from build123d import *

# Parameters (mm, degrees)
SKETCH1_W           = 15.8
SKETCH1_H           = 4
SKETCH1_W_2         = 2.7
SKETCH1_H_2         = 2.7
BOSS_EXTRUDE1_DEPTH = 7.65
SKETCH2_W           = 15.8
SKETCH2_H           = 4
SKETCH2_W_2         = 1.8
SKETCH2_H_2         = 1.8
BOSS_EXTRUDE2_DEPTH = 1
SKETCH3_W           = 2.45
SKETCH3_H           = 2.45
SKETCH3_W_2         = 1.8
SKETCH3_H_2         = 1.8
BOSS_EXTRUDE3_DEPTH = 6.35
SKETCH4_W           = 4.65
SKETCH4_H           = 0.65
SKETCH4_W_2         = 15.8
BOSS_EXTRUDE4_DEPTH = 1
SKETCH5_W           = 1
SKETCH5_H           = 1
SKETCH5_W_2         = 0.4
BOSS_EXTRUDE5_DEPTH = 2.5


with BuildPart() as part:
    # Sketch1 → Boss-Extrude1 (new body)
    with BuildSketch(Plane(origin=(0, 0, 0), x_dir=(1, 0, 0), z_dir=(0, 1, 0))):
        Rectangle(SKETCH1_W, SKETCH1_H)
        Rectangle(SKETCH1_W_2, SKETCH1_H_2, mode=Mode.SUBTRACT)
        with Locations((3, 0)):
            Rectangle(SKETCH1_W_2, SKETCH1_H_2, mode=Mode.SUBTRACT)
        with Locations((6, 0)):
            Rectangle(SKETCH1_W_2, SKETCH1_H_2, mode=Mode.SUBTRACT)
        with Locations((-6, 0)):
            Rectangle(SKETCH1_W_2, SKETCH1_H_2, mode=Mode.SUBTRACT)
        with Locations((-3, 0)):
            Rectangle(SKETCH1_W_2, SKETCH1_H_2, mode=Mode.SUBTRACT)
    extrude(amount=BOSS_EXTRUDE1_DEPTH)

    # Sketch2 → Boss-Extrude2 (add)
    with BuildSketch(Plane(origin=(0, 7.65, 0), x_dir=(1, 0, 0), z_dir=(0, 1, 0))):
        Rectangle(SKETCH2_W, SKETCH2_H)
        with Locations((-6, 0)):
            Rectangle(SKETCH2_W_2, SKETCH2_H_2, mode=Mode.SUBTRACT)
        with Locations((-3, 0)):
            Rectangle(SKETCH2_W_2, SKETCH2_H_2, mode=Mode.SUBTRACT)
        Rectangle(SKETCH2_W_2, SKETCH2_H_2, mode=Mode.SUBTRACT)
        with Locations((3, 0)):
            Rectangle(SKETCH2_W_2, SKETCH2_H_2, mode=Mode.SUBTRACT)
        with Locations((6, 0)):
            Rectangle(SKETCH2_W_2, SKETCH2_H_2, mode=Mode.SUBTRACT)
    extrude(amount=-BOSS_EXTRUDE2_DEPTH)

    # Sketch3 → Boss-Extrude3 (add)
    with BuildSketch(Plane(origin=(0, 7.65, 0), x_dir=(1, 0, 0), z_dir=(0, 1, 0))):
        with Locations((-6, 0)):
            Rectangle(SKETCH3_W, SKETCH3_H)
        with Locations((-6, 0)):
            Rectangle(SKETCH3_W_2, SKETCH3_H_2, mode=Mode.SUBTRACT)
        with Locations((-3, 0)):
            Rectangle(SKETCH3_W, SKETCH3_H)
        with Locations((-3, 0)):
            Rectangle(SKETCH3_W_2, SKETCH3_H_2, mode=Mode.SUBTRACT)
        Rectangle(SKETCH3_W, SKETCH3_H)
        Rectangle(SKETCH3_W_2, SKETCH3_H_2, mode=Mode.SUBTRACT)
        with Locations((3, 0)):
            Rectangle(SKETCH3_W, SKETCH3_H)
        with Locations((3, 0)):
            Rectangle(SKETCH3_W_2, SKETCH3_H_2, mode=Mode.SUBTRACT)
        with Locations((6, 0)):
            Rectangle(SKETCH3_W, SKETCH3_H)
        with Locations((6, 0)):
            Rectangle(SKETCH3_W_2, SKETCH3_H_2, mode=Mode.SUBTRACT)
    extrude(amount=BOSS_EXTRUDE3_DEPTH)

    # Sketch4 → Boss-Extrude4 (add)
    with BuildSketch(Plane.XZ):
        with Locations((-5.575, 2.325)):
            Rectangle(SKETCH4_W, SKETCH4_H)
        with Locations((5.575, 2.325)):
            Rectangle(SKETCH4_W, SKETCH4_H)
        with Locations((0, -2.325)):
            Rectangle(SKETCH4_W_2, SKETCH4_H)
    extrude(amount=-BOSS_EXTRUDE4_DEPTH)

    # Sketch5 → Boss-Extrude5 (add, symmetric)
    with BuildSketch(Plane(origin=(0, 0, 0), x_dir=(0, 0, -1), z_dir=(1, 0, 0))):
        Polygon((-3, 5.15), (-3, 6.15), (-3, 12.533692342), (-4, 13), (-4, 5.3), (-4, 1.5), (-3, 1.5), align=None)
        with Locations((-2.5, 5.65)):
            Rectangle(SKETCH5_W, SKETCH5_H)
        Polygon((-4.2, 1.5), (-4, 1.5), (-4, 5.3), (-4.2, 5.3), (-4.2, 2.5), align=None)
        with Locations((-4.4, 2)):
            Rectangle(SKETCH5_W_2, SKETCH5_H)
    extrude(amount=BOSS_EXTRUDE5_DEPTH, both=True)


solid = part.part
Can you work these out from the model? Positions are in its coordinate system, mm. A direction names the side the tool comes from. Round coordinates to 2 decimals unless told otherwise and drop trailing zeros. Order: outer loops, then holes, each group sorted by start corner. A loop starts at its lowest first (then second) coordinate and runs counter-clockwise, first axis right, second up. Notation, with made-up numbers: M 89,32 L 139,32 A28 ccw 139,70 Z; hole C 36,-22.75 d2. An arc over 180 degrees is marked long. Use a Markdown table: item, result.
1) Imagine slicing it at D-D (z = 0). Give the number of separate pieces and of enclosed holes in the cut face, then the cut area to 3 significant figures.
Geometry says:
| item | result |
|---|---|
| separate pieces | 6 |
| enclosed holes | 0 |
| area | 42.7 mm² |
2) I'm going to push flat-ended pins straight in: P1, Ø4, axis at x = 0, y = 4, coming from the -Z side; P2, Ø2.5, axis at x = -3, y = 10, coming from the -Z side (3 decimals); P3, Ø0.5, axis at x = -0.5, z = 2.5, coming from the +Y side. Where does each tip first touch, or does it pass through?
Geometry says:
| item | result |
|---|---|
| P1 | stops at z = -2 |
| P2 | stops at z = -1.225 |
| P3 | stops at y = 6.15 |
3) If we mould it in two halves opening along Z, with no side actions, what happens to faces 1 (the face through (-1.775, 11, 0)), 2 (the face through (6, 11, 1.225)), 3 (the face through (6, 3, -1.35))? For each: +Z half, -Z half, draft (parallel to the pull), parting line (faces both ways), or undercut.
Geometry says:
| item | result |
|---|---|
| face 1 | draft |
| face 2 | +Z half |
| face 3 | undercut |
4) On a 3-axis mill with a long thin cutter (end or side, diameter ignored), from which of +Z, -Z, +X, -X, +Y, -Y can I reach the whole of each face in a straight line? I mean faces 4 (the face through (-4.65, 3, 0)), 5 (the face through (4.775, 11, 0)), 6 (the face through (-3, 11, 1.225)), 7 (the face through (-6, 10, -0.9)), 8 (the face through (-1.225, 11, 0)). Say none if no direction works.
Geometry says:
| item | result |
|---|---|
| face 4 | -Y |
| face 5 | +Z, -Z, +Y |
| face 6 | +X, -X, +Y |
| face 7 | +Y, -Y |
| face 8 | -Z, +Y |
5) Imagine slicing it at A-A (y = 3.25). List the corners of the cut face in (x, z) for me, then the cut area to 4 significant figures.
Geometry says:
| item | result |
|---|---|
| outline | M -7.9,-2 L 7.9,-2 L 7.9,2 L -7.9,2 Z; M -2.5,3 L 2.5,3 L 2.5,4.2 L -2.5,4.2 Z; hole M -7.35,-1.35 L -4.65,-1.35 L -4.65,1.35 L -7.35,1.35 Z; hole M -4.35,-1.35 L -1.65,-1.35 L -1.65,1.35 L -4.35,1.35 Z; hole M -1.35,-1.35 L 1.35,-1.35 L 1.35,1.35 L -1.35,1.35 Z; hole M 1.65,-1.35 L 4.35,-1.35 L 4.35,1.35 L 1.65,1.35 Z; hole M 4.65,-1.35 L 7.35,-1.35 L 7.35,1.35 L 4.65,1.35 Z |
| area | 32.75 mm² |
6) If I drill on line 1 along X through (y, z) = (7, 0); line 2 along X through (y, z) = (3, -0.5); line 3 along Z through (x, y) = (-3, 11.5) (3 decimals), over which ranges is the centre line in solid material (lowest first)?
Geometry says:
| item | result |
|---|---|
| line 1 | x = -7.9 to -6.9, -5.1 to -3.9, -2.1 to -0.9, 0.9 to 2.1, 3.9 to 5.1, 6.9 to 7.9 |
| line 2 | x = -7.9 to -7.35, -4.65 to -4.35, -1.65 to -1.35, 1.35 to 1.65, 4.35 to 4.65, 7.35 to 7.9 |
| line 3 | z = -1.225 to -0.9, 0.9 to 1.225 |
7) Imagine slicing it at C-C (y = 5.5). List the corners of the cut face in (x, z) for me, then the cut area to 4 significant figures.
Geometry says:
| item | result |
|---|---|
| outline | M -7.9,-2 L 7.9,-2 L 7.9,2 L 2.5,2 L 2.5,4 L -2.5,4 L -2.5,2 L -7.9,2 Z; hole M -7.35,-1.35 L -4.65,-1.35 L -4.65,1.35 L -7.35,1.35 Z; hole M -4.35,-1.35 L -1.65,-1.35 L -1.65,1.35 L -4.35,1.35 Z; hole M -1.35,-1.35 L 1.35,-1.35 L 1.35,1.35 L -1.35,1.35 Z; hole M 1.65,-1.35 L 4.35,-1.35 L 4.35,1.35 L 1.65,1.35 Z; hole M 4.65,-1.35 L 7.35,-1.35 L 7.35,1.35 L 4.65,1.35 Z |
| area | 36.75 mm² |
8) Imagine slicing it at B-B (x = 5.5). List the corners of the cut face in (y, z) for me (3 decimals), then the cut area to 3 significant figures.
Geometry says:
| item | result |
|---|---|
| outline | M 0,-2.65 L 1,-2.65 L 1,-2 L 7.65,-2 L 7.65,-1.225 L 14,-1.225 L 14,-0.9 L 6.65,-0.9 L 6.65,-1.35 L 0,-1.35 Z; M 0,1.35 L 6.65,1.35 L 6.65,0.9 L 14,0.9 L 14,1.225 L 7.65,1.225 L 7.65,2 L 1,2 L 1,2.65 L 0,2.65 Z |
| area | 16.3 mm² |
